Autodesk Inventor part; units mm, degrees
ref_plane "YZ Plane" through (0, 0, 0) normal (1, 0, 0) x (0, 1, 0)
ref_plane "XZ Plane" through (0, 0, 0) normal (0, 1, 0) x (-1, 0, 0)
ref_plane "XY Plane" through (0, 0, 0) normal (0, 0, 1) x (1, 0, 0)
sketch "Sketch1" plane through (0, 0, 0) normal (0, 0, 1) x (1, 0, 0)
  line L0 (0, 0) -> (200, 0)
  line L1 (200, 0) -> (200, 125)
  line L2 (200, 125) -> (0, 125)
  line L3 (0, 125) -> (0, 0)
  dimension "d23" = 200
  dimension "d24" = 125
extrude "Extrusion1" add sketch "Sketch1" along normal blind 6.731
sketch "Sketch2" plane through (0, 0, 6.731) normal (0, 0, 1) x (1, 0, 0)
  line L0 (75.07, 105) -> (150, 105) construction
  line L1 (150, 105) -> (156.35, 105) construction
  line L2 (156.35, 105) -> (156.35, 56.74) construction
  line L3 (156.35, 56.74) -> (73.8, 56.74) construction
  line L4 (73.8, 56.74) -> (73.8, 105) construction
  line L5 (73.8, 105) -> (75.07, 105) construction
  line L6 (200, 0) -> (200, 125)
  line L7 (200, 125) -> (0, 125)
  dimension "d7" = 1.27
  dimension "d8" = 74.93
  dimension "d9" = 48.26
  dimension "d10" = 82.55
  dimension "d32" = 20
  dimension "d33" = 50
hole "Hole1" at (75.07, 105, 6.731) at (73.8, 56.74, 6.731) at (156.35, 56.74, 6.731) at (150, 105, 6.731) direction (0, 0, -1) diameter 3.176 end through all
sketch "Sketch3" plane through (0, 0, 6.731) normal (0, 0, 1) x (1, 0, 0)
  line L0 (200, 0) -> (200, 125)
  line L1 (0, 125) -> (0, 0)
  line L2 (0, 40) -> (6.731, 40)
  line L3 (6.731, 40) -> (6.731, 20)
  line L4 (6.731, 20) -> (0, 20)
  line L5 (0, 20) -> (0, 40)
  line L6 (200, 20) -> (193.269, 20)
  line L7 (193.269, 20) -> (193.269, 40)
  line L8 (193.269, 40) -> (200, 40)
  line L9 (200, 40) -> (200, 20)
  line L10 (0, 0) -> (200, 0)
  line L11 (0, 105) -> (6.731, 105)
  line L12 (6.731, 105) -> (6.731, 85)
  line L13 (6.731, 85) -> (0, 85)
  line L14 (0, 85) -> (0, 105)
  line L15 (200, 105) -> (193.269, 105)
  line L16 (193.269, 105) -> (193.269, 85)
  line L17 (193.269, 85) -> (200, 85)
  line L18 (200, 85) -> (200, 105)
  line L19 (90, 0) -> (110, 0)
  line L20 (110, 0) -> (110, 6.731)
  line L21 (110, 6.731) -> (90, 6.731)
  line L22 (90, 6.731) -> (90, 0)
  line L23 (200, 125) -> (0, 125)
  point P0 (100, 6.731)
  point P1 (100, 0)
  dimension "d19" = 6.731
  dimension "d20" = 20
  dimension "d25" = 20
  dimension "d28" = 20
extrude "Tabs" cut sketch "Sketch3" against normal up to next contours L6 L7 L8 L0 | L17 L16 L15 L0 | L1 L2 L3 L4 | L1 L11 L12 L13
sketch "Sketch4" plane through (0, 0, 6.731) normal (0, 0, 1) x (1, 0, 0)
  line L0 (0, 105) -> (6.731, 105)
  line L1 (0, 125) -> (90, 125)
  line L2 (90, 125) -> (90, 131.731)
  line L3 (90, 131.731) -> (0, 131.731)
  line L4 (0, 131.731) -> (0, 125)
  line L5 (200, 125) -> (110, 125)
  line L6 (110, 125) -> (110, 131.731)
  line L7 (110, 131.731) -> (200, 131.731)
  line L8 (200, 131.731) -> (200, 125)
  dimension "d29" = 20
extrude "Extrusion3" add sketch "Sketch4" against normal blind 6.731
equation "\"d0\" = THICKB"
equation "\"d19\" = THICKB"
equation "\"d21\" = THICKB"
equation "\"d30\" = THICKB"
equation "\"THICKA\" = 3.175"
equation "\"THICKB\" = 6.731"
equation "\"THICKC\" = 12.7"
equation "\"THICKPLY\" = 5"
equation "\"MAGDIA\" = 9.5"
equation "\"BALLDIA\" = 12"
properties part number "Controller_Base"
Here's how the part is built. I have some questions about the finished solid (model axes, mm). A direction names the side the tool comes from. Coordinates: 2 decimals unless noted, no trailing zeros. Order: outer loops, then holes, each group sorted by start corner. A loop starts at its lowest first (then second) coordinate and runs counter-clockwise, first axis right, second up.
1) Will these pins go through, and if not, where does the flat tip stop? pin 1 (2 mm diameter, centred on y = 52, z = 2.5, fed in from -X); pin 2 (3.5 mm diameter, centred on y = 94.5, z = 3, fed in from +X); pin 3 (2.5 mm diameter, centred on x = 75.07, y = 105, fed in from -Z); pin 4 (2 mm diameter, centred on x = 103.5, z = 2, fed in from +Y).
2) Imagine slicing it at B-B on x = 98. List the corners of the cut face in (y, z) for me, and give its area (3 significant figures).
3) Imagine slicing it at C-C on y = 23. List the corners of the cut face in (x, z) for me, and give its area (3 significant figures).
4) Imagine slicing it at A-A on z = 2.5. List the corners of the cut face in (x, y) for me, and give its area (3 significant figures).
5) I need wall thicknesses on line 1 (X direction, y = 56.74, z = 1.75); line 2 (Y direction, x = 73.8, z = 3.5); line 3 (Y direction, x = 91, z = 3.5). Which ranges of each line are inside material? Lowest first, please.
6) Which directions (+Z, -Z, +X, -X, +Y, -Y) give clear straight access to the entire face, cutting with the end or side of a thin tool? Please do faces 5 (the face through (90, 128, 3)), 6 (the face through (3, 40, 3)), 7 (the face through (193.269, 95, 3)).
7) We'd pull the mould along X, two halves only. Please class faces 1 (the face through (100, 125, 3)), 2 (the face through (6.731, 95, 3)), 3 (the face through (110, 128, 3)), 4 (the face through (99, 67, 6.731)): +X half, -X half, draft (parallel to the pull), parting line (faces both ways), or undercut.
Response values:
1. pin 1: stops at x = 0
1. pin 2: stops at x = 193.27
1. pin 3: passes through
1. pin 4: stops at y = 125
2. outline: (0, 0) - (125, 0) - (125, 6.73) - (0, 6.73) - close
2. area: 841 mm2
3. outline: (6.73, 0) - (193.27, 0) - (193.27, 6.73) - (6.73, 6.73) - close
3. area: 1,260 mm2
4. outline: (0, 0) - (200, 0) - (200, 20) - (193.27, 20) - (193.27, 40) - (200, 40) - (200, 85) - (193.27, 85) - (193.27, 105) - (200, 105) - (200, 131.73) - (110, 131.73) - (110, 125) - (90, 125) - (90, 131.73) - (0, 131.73) - (0, 105) - (6.73, 105) - (6.73, 85) - (0, 85) - (0, 40) - (6.73, 40) - (6.73, 20) - (0, 20) - close; hole circle Ø3.18 at (73.8, 56.74); hole circle Ø3.18 at (75.07, 105); hole circle Ø3.18 at (150, 105); hole circle Ø3.18 at (156.35, 56.74)
4. area: 25,600 mm2
5. line 1: x = 0 to 72.21, 75.39 to 154.76, 157.94 to 200
5. line 2: y = 0 to 55.15, 58.33 to 104.05, 105.95 to 131.73
5. line 3: y = 0 to 125
6. face 5: +Z, -Z, +Y
6. face 6: +Z, -Z, -X
6. face 7: +Z, -Z, +X
7. face 1: undercut
7. face 2: -X half
7. face 3: undercut
7. face 4: draft
